Could you check a few things on this model? Use its own coordinates, in mm. A direction names the side the tool comes from. Round coordinates to 2 decimals unless told otherwise and drop trailing zeros. Loops run counter-clockwise (first coordinate to the right, second up) from the corner with the lowest first, then second, coordinate; pieces in that order, holes last. Notation, with made-up numbers: (13.5, 44) -> (71.5, 44) arc R23 ccw to (71.5, 65) -> close; hole circle Ø10 at (74, 33.25). An arc over 180 degrees is marked (long way). One line per item, written item: value.
```python
from build123d import *

# Parameters (mm, degrees)
BOSS_EXTRUDE1_DEPTH             = 50.8
BOTTOMCOVERSKETCH3_W            = 66
BOTTOMCOVERSKETCH3_H            = 2
BOTTOMCOVERBOSS_EXTRUDE2_DEPTH  = 70
MOUNTINGHOLESSKETCH4_R          = 2.05
MOUNTINGHOLESCUT_EXTRUDE2_DEPTH = 4
CABLEHOLECUT_EXTRUDE1_REACH     = 118.639


with BuildPart() as part:
    # Sketch1 → Boss-Extrude1 (new body)
    with BuildSketch(Plane(origin=(0, 0, 0), x_dir=(1, 0, 0), z_dir=(0, 1, 0))):
        Polygon((-10, 0), (0, 0), (0, 68), (70, 68), (70, 0), (80, 0), (80, -4), (68, -4), (68, 66), (2, 66), (2, -4), (-10, -4), align=None)
    extrude(amount=BOSS_EXTRUDE1_DEPTH)

    # BottomCoverSketch3 → BottomCoverBoss-Extrude2 (add)
    with BuildSketch(Plane.XY.offset(-66)):
        with Locations((35, 1)):
            Rectangle(BOTTOMCOVERSKETCH3_W, BOTTOMCOVERSKETCH3_H)
    extrude(amount=BOTTOMCOVERBOSS_EXTRUDE2_DEPTH)

    # MountingHolesSketch4 → MountingHolesCut-Extrude2 (cut)
    with BuildSketch(Plane.XY.offset(4)):
        with Locations((74, 25.4)):
            Circle(MOUNTINGHOLESSKETCH4_R)
        with Locations((-4, 25.4)):
            Circle(MOUNTINGHOLESSKETCH4_R)
    extrude(amount=-MOUNTINGHOLESCUT_EXTRUDE2_DEPTH, mode=Mode.SUBTRACT)

    # CableHoleSketch2 → CableHoleCut-Extrude1 (cut, up to next)
    with BuildSketch(Plane(origin=(70, 0, 0), x_dir=(0, 0, -1), z_dir=(1, 0, 0)), mode=Mode.PRIVATE) as cableholecut_extrude1_sk1:
        with BuildLine():
            Line((30.5, 50.8), (35.5, 50.8))
            add(Edge.make_bspline(
                [(35.193240855, 47.440356377), (35.5, 49.010381841), (35.5, 50.8)],
                knots=[1.070199647, 1.070199647, 1.070199647, 1.570796327, 1.570796327, 1.570796327], degree=2, weights=[1, 0.968838568, 1]))
            ThreePointArc((35.193240855, 47.440356377), (33, 39.55), (30.806759145, 47.440356377))
            add(Edge.make_bspline(
                [(30.5, 50.8), (30.5, 49.010381841), (30.806759145, 47.440356377)],
                knots=[4.71238898, 4.71238898, 4.71238898, 5.21298566, 5.21298566, 5.21298566], degree=2, weights=[1, 0.968838568, 1]))
        make_face()
    cableholecut_extrude1_tool1 = extrude(cableholecut_extrude1_sk1.sketch, amount=-CABLEHOLECUT_EXTRUDE1_REACH, mode=Mode.PRIVATE) & part.part
    add(cableholecut_extrude1_tool1.solids().sort_by_distance((70, 44.916526, -33))[0], mode=Mode.SUBTRACT)


solid = part.part
```
Item 1: If we section it at A-A on y = 43.8: List the corners of the cut face in (x, z) for me.
Output:
outline: (-10, 0) -> (0, 0) -> (0, -68) -> (70, -68) -> (70, -37.25) -> (68, -37.25) -> (68, -66) -> (2, -66) -> (2, 4) -> (-10, 4) -> close; (68, -28.75) -> (70, -28.75) -> (70, 0) -> (80, 0) -> (80, 4) -> (68, 4) -> close
Item 2: If we mould it in two halves opening along X, with no side actions, what happens to faces 1 (the face through (69.6, 50.8, -6.9)), 2 (the face through (35, 2, -31)), 3 (the face through (35, 26, -66)), 4 (the face through (70, 25, -34))? For each: released by +X, released by -X, zero draft, split by the parting line, or undercut.
Output:
face 1: zero draft
face 2: undercut
face 3: undercut
face 4: released by +X
Item 3: For faces 5 (the face through (0, 25, -34)), 6 (the face through (68, 26, -31)), 7 (the face through (69.014, 39.553, -33.155)), 8 (the face through (77, 25, 0)), 9 (the face through (80, 25, 2)), which set-ups out of +Z, -Z, +X, -X, +Y, -Y let a thin tool reach every point of the face, with its end or its side?
Output:
face 5: -Z, -X, +Y, -Y
face 6: +Z, +Y
face 7: +X
face 8: -Z, +X, +Y, -Y
face 9: +Z, -Z, +X, +Y, -Y
Item 4: If we section it at C-C on z = -18: List the corners of the cut face in (x, y) for me.
Output:
outline: (0, 0) -> (70, 0) -> (70, 50.8) -> (68, 50.8) -> (68, 2) -> (2, 2) -> (2, 50.8) -> (0, 50.8) -> close
Item 5: If we section it at B-B on x = -4: List the corners of the cut face in (y, z) for me.
Output:
outline: (0, 0) -> (23.35, 0) -> (23.35, 4) -> (0, 4) -> close; (27.45, 0) -> (50.8, 0) -> (50.8, 4) -> (27.45, 4) -> close
Item 6: If we section it at D-D on y = 25.4: List the corners of the cut face in (x, z) for me.
Output:
outline: (-10, 0) -> (-6.05, 0) -> (-6.05, 4) -> (-10, 4) -> close; (-1.95, 0) -> (0, 0) -> (0, -68) -> (70, -68) -> (70, 0) -> (71.95, 0) -> (71.95, 4) -> (68, 4) -> (68, -66) -> (2, -66) -> (2, 4) -> (-1.95, 4) -> close; (76.05, 0) -> (80, 0) -> (80, 4) -> (76.05, 4) -> close
Item 7: Will these pins go through, and if not, where does the flat tip stop? pin 1 Ø1 at (y, z) = (26, -41.5) entering from -X; pin 2 Ø4.5 at (x, y) = (-4, 25.4) entering from -Z; pin 3 Ø8 at (y, z) = (31.5, -27) entering from +X; pin 4 Ø3.5 at (x, y) = (74, 25.4) entering from -Z.
Output:
pin 1: stops at x = 0
pin 2: stops at z = 0
pin 3: stops at x = 70
pin 4: passes through
Item 8: I need wall thicknesses on line 1 (X direction, y = 31, z = -43.5); line 2 (Y direction, x = -4, z = 2.65); line 3 (Z direction, x = 18.5, y = 20.5). Which ranges of each line are inside material? Lowest first, please. Write a range as from..to.
Output:
line 1: x = 0..2, 68..70
line 2: y = 0..23.35, 27.45..50.8
line 3: z = -68..-66
